Here's how the part is built. I have some questions about the finished solid (model axes, mm). Face numbers are marked on the shaded views. A direction names the side the tool comes from. Coordinates: 2 decimals unless noted, no trailing zeros. Order: outer loops, then holes, each group sorted by start corner. A loop starts at its lowest first (then second) coordinate and runs counter-clockwise, first axis right, second up. Notation, with made-up numbers: (36.25, 18.25) -> (72.25, 18.25) arc R17 cw to (72.25, 25.25) -> close; hole circle Ø1 at (9.5, 62.5). An arc over 180 degrees is marked (long way). One line per item, written item: value. Start each with the question number.
```python
from build123d import *

# Parameters (mm, degrees)
BOSS_EXTRUDE1_DEPTH = 0.75
BOSS_EXTRUDE2_DEPTH = 20


with BuildPart() as part:
    # Sketch1 → Boss-Extrude1 (new, symmetric)
    with BuildSketch(Plane(origin=(0, 0, 0), x_dir=(1, 0, 0), z_dir=(0, 1, 0))):
        with BuildLine():
            Line((-28.307864731, 69.452608262), (-13, 32.496153619))
            Line((-13, 32.496153619), (13, 32.496153619))
            Line((13, 32.496153619), (28.307864731, 69.452608262))
            ThreePointArc((28.307864731, 69.452608262), (0, 75), (-28.307864731, 69.452608262))
        make_face()
        with BuildLine():
            Line((-4.543006128, 56.502305121), (-1.89666405, 50.113470186))
            ThreePointArc((-1.89666405, 50.113470186), (-1.52835475, 49.664684006), (-0.972784517, 49.496153619))
            Line((-0.972784517, 49.496153619), (0.972784517, 49.496153619))
            ThreePointArc((0.972784517, 49.496153619), (1.52835475, 49.664684006), (1.89666405, 50.113470186))
            Line((1.89666405, 50.113470186), (4.543006128, 56.502305121))
            ThreePointArc((4.543006128, 56.502305121), (4.467823117, 57.413868704), (3.682620044, 57.882970808))
            ThreePointArc((3.682620044, 57.882970808), (0, 58), (-3.682620044, 57.882970808))
            ThreePointArc((-3.682620044, 57.882970808), (-4.467823117, 57.413868704), (-4.543006128, 56.502305121))
        make_face(mode=Mode.SUBTRACT)
    boss_extrude1 = extrude(amount=BOSS_EXTRUDE1_DEPTH, both=True)

    # Sketch2 → Boss-Extrude2 (add)
    with BuildSketch(Plane.XZ.offset(0.75)):
        with BuildLine():
            Line((-0.972784517, -47.996153619), (0.972784517, -47.996153619))
            ThreePointArc((0.972784517, -47.996153619), (2.3617101, -48.417479588), (3.282483349, -49.539445038))
            Line((3.282483349, -49.539445038), (5.928825426, -55.928279972))
            ThreePointArc((5.928825426, -55.928279972), (5.7408679, -58.207188929), (3.777860218, -59.379944191))
            ThreePointArc((3.777860218, -59.379944191), (0, -59.5), (-3.777860218, -59.379944191))
            ThreePointArc((-3.777860218, -59.379944191), (-5.7408679, -58.207188929), (-5.928825426, -55.928279972))
            Line((-5.928825426, -55.928279972), (-3.282483349, -49.539445038))
            ThreePointArc((-3.282483349, -49.539445038), (-2.3617101, -48.417479588), (-0.972784517, -47.996153619))
        make_face()
        with BuildLine():
            Line((1.89666405, -50.113470186), (4.543006128, -56.502305121))
            ThreePointArc((4.543006128, -56.502305121), (4.467823117, -57.413868704), (3.682620044, -57.882970808))
            ThreePointArc((3.682620044, -57.882970808), (0, -58), (-3.682620044, -57.882970808))
            ThreePointArc((-3.682620044, -57.882970808), (-4.467823117, -57.413868704), (-4.543006128, -56.502305121))
            Line((-4.543006128, -56.502305121), (-1.89666405, -50.113470186))
            ThreePointArc((-1.89666405, -50.113470186), (-1.52835475, -49.664684006), (-0.972784517, -49.496153619))
            Line((-0.972784517, -49.496153619), (0.972784517, -49.496153619))
            ThreePointArc((0.972784517, -49.496153619), (1.52835475, -49.664684006), (1.89666405, -50.113470186))
        make_face(mode=Mode.SUBTRACT)
    extrude(amount=BOSS_EXTRUDE2_DEPTH)

    # Mirror1: Boss-Extrude1 across plane
    add(boss_extrude1.mirror(Plane(origin=(0, -10.75, 0), x_dir=(0, 0, 1), z_dir=(0, -1, 0))))


solid = part.part
```
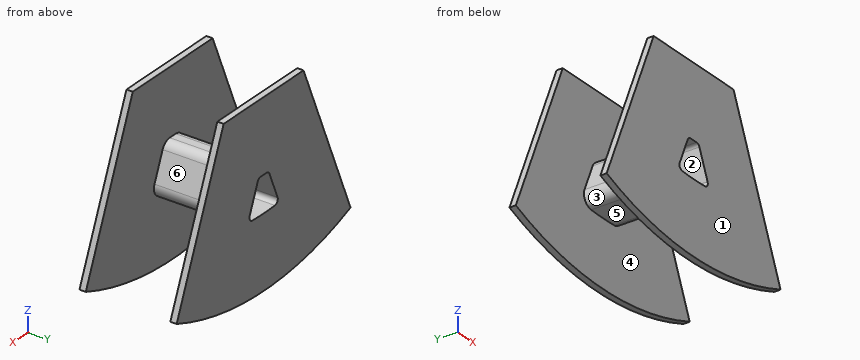
Q1. For P1, Ø6, axis at y = -19.5, z = -44.5, coming from the -X side; P2, Ø8, axis at y = -3, z = -66, coming from the +X side; P3, Ø8, axis at x = 3, y = -2, coming from the +Z side; P4, Ø1, axis at y = -8.5, z = -51.5, coming from the +X side, each with a flat end and sliding along its axis, tell me the tip position at first contact or that it passes through.
Q2. If we mould it in two halves opening along Y, with no side actions, what happens to the marked faces 1, 2 and 3? For each: +Y half, -Y half, draft (parallel to the pull), parting line (faces both ways), or undercut.
Q3. For the marked faces 4, 5 and 6, which set-ups out of +Z, -Z, +X, -X, +Y, -Y let a thin tool reach every point of the face, with its end or its side?
Q4. Imagine slicing it at C-C (x = -25). Write out the boundary of the cut face in (y, z).
Q5. I need wall thicknesses on line 1 (Y direction, x = -15, z = -69); line 2 (X direction, y = -11, z = -51); line 3 (X direction, y = -2, z = -55.5). Which ranges of each line are inside material? Lowest first, please.
Q6. Imagine slicing it at D-D (z = -65.5). Write out the boundary of the cut face in (x, y).
Q7. Imagine slicing it at B-B (y = -4.25). Write out the boundary of the cut face in (x, z).
Q8. Imagine slicing it at A-A (z = -51.5). Write out the boundary of the cut face in (x, y), plus the area to 3 significant figures.
Completed:
1. P1: stops at x = -19.1
1. P2: stops at x = 28.25
1. P3: stops at z = -32.5
1. P4: stops at x = 4.3
2. face 1: -Y half
2. face 2: draft
2. face 3: undercut
3. face 4: none
3. face 5: -Z
3. face 6: +Z, +X
4. outline: (-22.25, -70.71) -> (-20.75, -70.71) -> (-20.75, -61.47) -> (-22.25, -61.47) -> close; (-0.75, -70.71) -> (0.75, -70.71) -> (0.75, -61.47) -> (-0.75, -61.47) -> close
5. line 1: y = -22.25 to -20.75, -0.75 to 0.75
5. line 2: x = -3.89 to -2.26, 2.26 to 3.89
5. line 3: x = -5.75 to -4.13, 4.13 to 5.75
6. outline: (-26.67, -22.25) -> (26.67, -22.25) -> (26.67, -20.75) -> (-26.67, -20.75) -> close; (-26.67, -0.75) -> (26.67, -0.75) -> (26.67, 0.75) -> (-26.67, 0.75) -> close
7. outline: (-5.93, -55.93) arc R2.5 ccw to (-3.78, -59.38) arc R59.5 ccw to (3.78, -59.38) arc R2.5 ccw to (5.93, -55.93) -> (3.28, -49.54) arc R2.5 ccw to (0.97, -48) -> (-0.97, -48) arc R2.5 ccw to (-3.28, -49.54) -> close; hole (-4.54, -56.5) arc R1 ccw to (-3.68, -57.88) arc R58 ccw to (3.68, -57.88) arc R1 ccw to (4.54, -56.5) -> (1.9, -50.11) arc R1 ccw to (0.97, -49.5) -> (-0.97, -49.5) arc R1 ccw to (-1.9, -50.11) -> close
8. outline: (-20.87, -22.25) -> (-2.47, -22.25) -> (-2.47, 0.75) -> (-20.87, 0.75) -> (-20.87, -0.75) -> (-4.09, -0.75) -> (-4.09, -20.75) -> (-20.87, -20.75) -> close; (2.47, -22.25) -> (20.87, -22.25) -> (20.87, -20.75) -> (4.09, -20.75) -> (4.09, -0.75) -> (20.87, -0.75) -> (20.87, 0.75) -> (2.47, 0.75) -> close
8. area: 175 mm2
